CAD build for the part. Positions are in the model's coordinates, mm. A direction names the side the tool comes from. Round coordinates to 2 decimals unless told otherwise and drop trailing zeros. Loops run counter-clockwise (first coordinate to the right, second up) from the corner with the lowest first, then second, coordinate; pieces in that order, holes last. Notation, with made-up numbers: M 33,-28 L 38,-28 A21 cw 38,-3 Z; hole C -34,35 d6. An arc over 180 degrees is marked long. Put each result on its own line as item: value. Start each with the question number.
from build123d import *

# Parameters (mm, degrees)
F1_DEPTH = 4
F2_DEPTH = 38
F3_R     = 1


with BuildPart() as f1:
    # F0 (on Top) → F1 (new body)
    with BuildSketch(Plane.XY):
        Polygon((0, 20.327126), (0, 0), (0, -20.327126), (0, -65.713919), (12.5, -65.713919), (16.5, -65.713919), (16.5, -62), (16.5, -58.286081), (12.5, -58.286081), (12.5, -62), (4.5, -62), (4.5, 0), (4.5, 62), (12.5, 62), (12.5, 58.286081), (16.5, 58.286081), (16.5, 62), (16.5, 65.713919), (12.5, 65.713919), (0, 65.713919), align=None)
        Polygon((0, -20.327126), (0, 0), (0, 20.327126), (-5.289079, 20.327126), (-7, 24.327126), (-9, 24.327126), (-9, 0), (-9, -24.327126), (-7, -24.327126), (-5.289079, -20.327126), align=None)
    extrude(amount=-F1_DEPTH)

    # F0 (on Top) → F2 (join)
    with BuildSketch(Plane.XY):
        Polygon((0, -20.327126), (0, 0), (0, 20.327126), (-5.289079, 20.327126), (-7, 24.327126), (-9, 24.327126), (-9, 0), (-9, -24.327126), (-7, -24.327126), (-5.289079, -20.327126), align=None)
        Polygon((0, 20.327126), (0, 0), (0, -20.327126), (0, -65.713919), (12.5, -65.713919), (16.5, -65.713919), (16.5, -62), (16.5, -58.286081), (12.5, -58.286081), (12.5, -62), (4.5, -62), (4.5, 0), (4.5, 62), (12.5, 62), (12.5, 58.286081), (16.5, 58.286081), (16.5, 62), (16.5, 65.713919), (12.5, 65.713919), (0, 65.713919), align=None)
    extrude(amount=-F2_DEPTH)

    # F3
    f3_edges = [f1.edges().sort_by_distance(p)[0] for p in [
        (0, -43.020523, 0),
        (8.25, -65.713919, 0),
        (16.5, -62, 0),
        (14.5, -58.286081, 0),
        (12.5, -60.143041, 0),
        (8.5, -62, 0),
        (4.5, 0, 0),
        (8.5, 62, 0),
        (12.5, 60.143041, 0),
        (14.5, 58.286081, 0),
        (16.5, 62, 0),
        (8.25, 65.713919, 0),
        (0, 43.020523, 0),
        (-2.64454, 20.327126, 0),
        (-6.14454, 22.327126, 0),
        (-8, 24.327126, 0),
        (-9, 0, 0),
        (-8, -24.327126, 0),
        (-6.14454, -22.327126, 0),
        (-2.64454, -20.327126, 0),
        (8.25, -65.713919, -38),
        (16.5, -62, -38),
        (14.5, -58.286081, -38),
        (12.5, -60.143041, -38),
        (8.5, -62, -38),
        (4.5, 0, -38),
        (8.5, 62, -38),
        (12.5, 60.143041, -38),
        (14.5, 58.286081, -38),
        (16.5, 62, -38),
        (8.25, 65.713919, -38),
        (0, 43.020523, -38),
        (-2.64454, 20.327126, -38),
        (-6.14454, 22.327126, -38),
        (-8, 24.327126, -38),
        (-9, 0, -38),
        (-8, -24.327126, -38),
        (-6.14454, -22.327126, -38),
        (-2.64454, -20.327126, -38),
        (0, -43.020523, -38),
        (16.5, -58.286081, -19),
        (12.5, -58.286081, -19),
        (12.5, 58.286081, -19),
        (16.5, 58.286081, -19),
        (-9, 24.327126, -19),
        (-9, -24.327126, -19),
        (16.5, 65.713919, -19),
        (0, 65.713919, -19),
        (0, -65.713919, -19),
        (16.5, -65.713919, -19),
    ]]
    fillet(f3_edges, radius=F3_R)


solid = f1.part
(1) Cut at A-A on x = 6.5. List the corners of the cut face in (y, z), and give its area (3 significant figures).
(2) Cut at C-C on x = -3.5. List the corners of the cut face in (y, z), and give its area (3 significant figures).
(3) Drill centre lines: line 1 along Y through (x, z) = (5.5, -23); line 2 along Y through (x, z) = (15.25, -16.5); line 3 along X through (y, z) = (-31, -27.5). Where is each one in solid material? Low to high.
(4) Tool access for faces 1 (the cylindrical face through (-6.305, 21.938, -0.285)), 2 (the flat face through (-6.16, -22.36, -18.75)), 3 (the cylindrical face through (-6.277, -21.873, -0.285)), 4 (the flat face through (9, -62, -19)), 5 (the flat face through (-3, 20.327, -19)): list every direction of +Z, -Z, +X, -X, +Y, -Y with a clear straight run to the whole face (end or side of a thin tool).
(5) Cut at B-B on y = -29. List the corners of the cut face in (x, z), and give its area (3 significant figures).
(6) Flat gauge pins, fed straight in: pin 1 Ø4 at (x, z) = (-2.5, -27) entering from -Y; pin 2 Ø1 at (y, z) = (32, -21) entering from +X; pin 3 Ø11 at (y, z) = (41.5, -15) entering from -X. Where does each tip first touch, or does it go through?
(7) Mould opens along Y. For faces 6 (the flat face through (-6.133, 22.299, -18.748)), 7 (the flat face through (8, 62, -19)), 8 (the flat face through (0, 43, -19)), 9 (the cylindrical face through (-6.263, -21.879, -37.699)) say: +Y half, -Y half, draft (parallel to the pull), parting line (faces both ways), or undercut.
Taken from the geometry:
1. outline: M -65.71,-37 A1 ccw -64.71,-38 L -63,-38 A1 ccw -62,-37 L -62,-1 A1 ccw -63,0 L -64.71,0 A1 ccw -65.71,-1 Z; M 62,-37 A1 ccw 63,-38 L 64.71,-38 A1 ccw 65.71,-37 L 65.71,-1 A1 ccw 64.71,0 L 63,0 A1 ccw 62,-1 Z
1. area: 281 mm2
2. outline: M -20.33,-37 A1 ccw -19.33,-38 L 19.33,-38 A1 ccw 20.33,-37 L 20.33,-1 A1 ccw 19.33,0 L -19.33,0 A1 ccw -20.33,-1 Z
2. area: 1,540 mm2
3. line 1: -65.71 to -62, 62 to 65.71
3. line 2: -65.71 to -58.29, 58.29 to 65.71
3. line 3: 0 to 4.5
4. face 1: +Z, +Y
4. face 2: +Z, -Z, -Y
4. face 3: +Z, -Y
4. face 4: +Z, -Z
4. face 5: +Z, -Z, +Y
5. outline: M 0,-37 A1 ccw 1,-38 L 3.5,-38 A1 ccw 4.5,-37 L 4.5,-1 A1 ccw 3.5,0 L 1,0 A1 ccw 0,-1 Z
5. area: 170 mm2
6. pin 1: y = -20.33
6. pin 2: x = 4.5
6. pin 3: x = 0
7. face 6: +Y half
7. face 7: undercut
7. face 8: draft
7. face 9: -Y half
